The listing builds one solid part. Answer for the finished solid, in the listing's coordinates (mm). Face numbers are marked on the shaded views. A direction names the side the tool comes from. Give positions to 0.01 mm unless a question says otherwise; leave off trailing zeros. Loops run counter-clockwise (first coordinate to the right, second up) from the corner with the lowest first, then second, coordinate; pieces in that order, holes last. Notation, with made-up numbers: M 8,-10 L 43,-10 A20 ccw 43,24 Z; hole C 15.25,-30 d4. An arc over 180 degrees is marked long. Use one line per item in the form item = value. Start each with the question number.
1. Straight lines are drawn through the part: line 1 (Z direction, x = 15, y = 9.5); line 2 (X direction, y = -3, z = -9.25); line 3 (Y direction, x = 1, z = -3.5). For each, find the intervals that lie inside material, in ascending order. Write a range as from..to.
2. For the marked faces 1 and 2, determine the directions among +Z, -Z, +X, -X, +Y, -Y from which every point of the face is accessible in a straight line to the end or side of a thin tool.
3. The part is cut by section C-C (y = -10.5). Write down the section's boundary in (x, z), and give its area (3 significant figures).
4. The part is cut by section B-B (x = 0). Write down the section's boundary in (y, z).
5. Each of these flat-tipped pins is pushed along its axis until it touches: pin 1 Ø6 at (x, z) = (5, 0.5) entering from +Y; pin 2 Ø3 at (x, y) = (-22.53, 0) entering from -Z; pin 3 Ø5.5 at (x, y) = (22.53, 0) entering from -Z; pin 4 Ø6 at (x, y) = (-8, 19.5) entering from -Z. Where does it stop, or does it pass through?
6. The part is cut by section D-D (y = 8.5). Write down the section's boundary in (x, z).
7. The part is cut by section A-A (y = 0). Write down the section's boundary in (x, z), and give its area (3 significant figures).
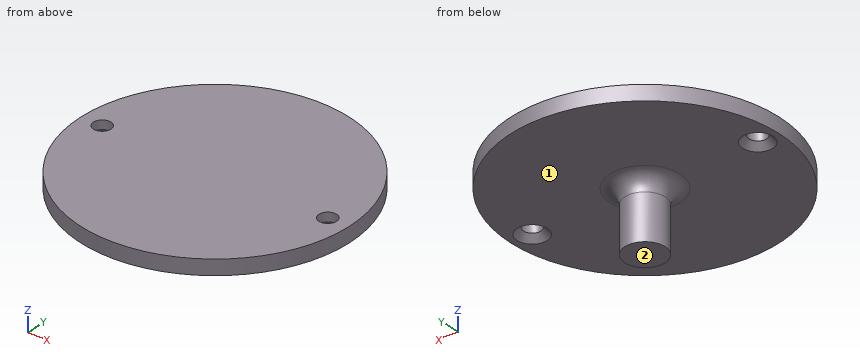
Autodesk Fusion 360 part; units mm, degrees
sketch "Sketch1" plane through (0, 0, 0) normal (0, 0, 1) x (1, 0, 0)
  circle A0 centre (0, 0) radius 26.7785
  line L0 (0, 0) -> (-26.7785, 0) construction
  line L1 (0, 0) -> (26.7785, 0) construction
  circle A1 centre (-22.5285, 0) radius 3
  circle A2 centre (-22.5285, 0) radius 1.75
  circle A3 centre (22.5285, 0) radius 3
  circle A4 centre (22.5285, 0) radius 1.75
  circle A5 centre (0, 0) radius 4
  dimension "d1" = 53.557
  dimension "d2" = 6
  dimension "d3" = 3.5
  dimension "d4" = 4.25
  dimension "d5" = 6
  dimension "d6" = 3.5
  dimension "d8" = 4.25
  dimension "d12" = 8
extrude "Extrude1" add sketch "Sketch1" along normal blind 3 contours A0 | A1 | A3 | A5
chamfer "Chamfer1" distance 1.25 angle 45 2 edges at (20.8969, 0.6328, 0) (-24.1601, 0.6328, 0)
extrude "Extrude2" add sketch "Sketch1" against normal blind 12 contours A5
fillet "Fillet1" radius 3 1 edges at (-3.7293, -1.4465, 0)
Derived:
q1.line_1 = 0..3
q1.line_2 = -2.65..2.65
q1.line_3 = -3.87..3.87
q2.face_1 = -Z
q2.face_2 = -Z, +X, -X, +Y, -Y
q3.outline = M -24.63,0 L 24.63,0 L 24.63,3 L -24.63,3 Z
q3.area = 148 mm2
q4.outline = M -26.78,0 L -7,0 A3 cw -4,-3 L -4,-12 L 4,-12 L 4,-3 A3 cw 7,0 L 26.78,0 L 26.78,3 L -26.78,3 Z
q5.pin_1 = 26.7
q5.pin_2 = through
q5.pin_3 = 0.25
q5.pin_4 = 0
q6.outline = M -25.39,0 L 25.39,0 L 25.39,3 L -25.39,3 Z
q7.outline = M -26.78,0 L -25.53,0 L -24.28,1.25 L -24.28,3 L -26.78,3 Z; M -20.78,1.25 L -19.53,0 L -7,0 A3 cw -4,-3 L -4,-12 L 4,-12 L 4,-3 A3 cw 7,0 L 19.53,0 L 20.78,1.25 L 20.78,3 L -20.78,3 Z; M 24.28,1.25 L 25.53,0 L 26.78,0 L 26.78,3 L 24.28,3 Z
q7.area = 236 mm2
